from build123d import *

# Parameters (mm, degrees)
F0_W     = 25
F0_H     = 25
F1_DEPTH = 110
F2_W     = 27.421856
F2_H     = 90
F3_DEPTH = 20
F4_R     = 3.25
F5_DEPTH = 110.001


with BuildPart() as f1:
    # F0 (on Top) → F1 (new body)
    with BuildSketch(Plane.XY):
        with Locations((-25.848038, 19.508659)):
            Rectangle(F0_W, F0_H)
    extrude(amount=F1_DEPTH)

    # F2 (on face) → F3 (cut)
    with BuildSketch(Plane.XZ.offset(-7.008659)):
        with Locations((-32.058966, 55)):
            Rectangle(F2_W, F2_H)
    extrude(amount=-F3_DEPTH, mode=Mode.SUBTRACT)

    # F4 (on face) → F5 (cut, through all)
    with BuildSketch(Plane.XY.offset(110)):
        with Locations((-25.848038, 19.508659)):
            Circle(F4_R)
    extrude(amount=-F5_DEPTH, mode=Mode.SUBTRACT)


solid = f1.part
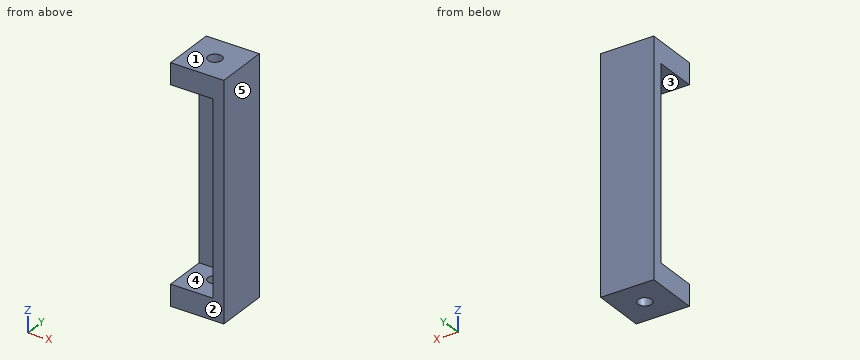
For this review, take the finished solid that the model builds, in its own axes (mm). Face numbers are marked on the shaded views. A direction names the side the tool comes from. Round coordinates to 2 decimals unless told otherwise and drop trailing zeros. Order: outer loops, then holes, each group sorted by start corner. A loop starts at its lowest first (then second) coordinate and runs counter-clockwise, first axis right, second up. Notation, with made-up numbers: (55, 74) -> (111, 74) arc R21 ccw to (111, 94) -> close; hole circle Ø6 at (33, -37). An arc over 180 degrees is marked (long way). Write item = value, one per line. Start each with the question number.
1) Take a section at C-C on z = 21. State the section outline as (x, y) points.
2) The part is to be moulded in two halves that separate along Z. For the marked faces 1, 2 and 3, say which applies: +Z half, -Z half, draft (parallel to the pull), parting line (faces both ways), or undercut.
3) Tool access review of the marked faces 4 and 5: name each direction out of +Z, -Z, +X, -X, +Y, -Y from which nothing blocks a thin tool from reaching the whole face with its end or side.
4) Take a section at D-D on x = -35. State the section outline as (y, z) points.
5) To check wall thickness, follow line 1 (Z direction, x = -36.25, y = 23.25); line 2 (Y direction, x = -27.5, z = 54.5); line 3 (X direction, y = 15.75, z = 86.5). State the ranges of each line that lie inside material, in increasing order. Write a range as from..to.
6) Take a section at B-B on x = -27.75. State the section outline as (y, z) points, plus the area to 3 significant figures.
7) Take a section at A-A on y = 20.5. State the section outline as (x, z) points, plus the area to 3 significant figures.
8) Insertion check: pin 1 (2 mm diameter, centred on x = -21, z = 29.5, fed in from -Y). The pin has a flat end and moves straight along its axis. Give the tip position at first contact, or say it passes through.
Verdict:
q1.outline = (-38.35, 27.01) -> (-18.35, 27.01) -> (-18.35, 7.01) -> (-13.35, 7.01) -> (-13.35, 32.01) -> (-38.35, 32.01) -> close
q2.face_1 = +Z half
q2.face_2 = draft
q2.face_3 = undercut
q3.face_4 = -X, -Y
q3.face_5 = +Z, -Z, +X, +Y, -Y
q4.outline = (7.01, 0) -> (32.01, 0) -> (32.01, 110) -> (7.01, 110) -> (7.01, 100) -> (27.01, 100) -> (27.01, 10) -> (7.01, 10) -> close
q5.line_1 = 0..10, 100..110
q5.line_2 = 27.01..32.01
q5.line_3 = -18.35..-13.35
q6.outline = (7.01, 0) -> (16.87, 0) -> (16.87, 10) -> (7.01, 10) -> close; (7.01, 100) -> (16.87, 100) -> (16.87, 110) -> (7.01, 110) -> close; (22.14, 0) -> (32.01, 0) -> (32.01, 110) -> (22.14, 110) -> (22.14, 100) -> (27.01, 100) -> (27.01, 10) -> (22.14, 10) -> close
q6.area = 845 mm2
q7.outline = (-38.35, 0) -> (-28.94, 0) -> (-28.94, 10) -> (-38.35, 10) -> close; (-38.35, 100) -> (-28.94, 100) -> (-28.94, 110) -> (-38.35, 110) -> close; (-22.75, 0) -> (-13.35, 0) -> (-13.35, 110) -> (-22.75, 110) -> (-22.75, 100) -> (-18.35, 100) -> (-18.35, 10) -> (-22.75, 10) -> close
q7.area = 826 mm2
q8.pin_1 = 27.01
